Verification items for the finished model (mm, model axes). A direction names the side the tool comes from. Round coordinates to 2 decimals unless told otherwise and drop trailing zeros. Loops run counter-clockwise (first coordinate to the right, second up) from the corner with the lowest first, then second, coordinate; pieces in that order, holes last. Notation, with made-up numbers: (-3, 55) -> (20, 55) arc R36 ccw to (20, 91) -> close; hole circle Ø4 at (1, 25). An arc over 180 degrees is marked (long way). Write item = value, one per line. Start each with the question number.
```python
from build123d import *

# Parameters (mm, degrees)
F0_W     = 57.15
F0_H     = 44.45
F1_DEPTH = 25.4
F3_DEPTH = 12.7
F4_DEPTH = 19.05


with BuildPart() as f1:
    # F0 (on Front) → F1 (new body)
    with BuildSketch(Plane.XZ):
        with Locations((28.575, 22.225)):
            Rectangle(F0_W, F0_H)
    extrude(amount=F1_DEPTH)

    # F2 (on face) → F3 (cut)
    with BuildSketch(Plane.XZ.offset(25.4)):
        with BuildLine():
            Line((57.15, 44.45), (19.05, 44.45))
            Line((19.05, 44.45), (24.390971, 35.103302))
            ThreePointArc((24.390971, 35.103302), (41.651297, 30.339378), (36.992666, 13.050335))
            Line((36.992666, 13.050335), (44.45, 0))
            Line((44.45, 0), (57.15, 0))
            Line((57.15, 0), (57.15, 44.45))
        make_face()
    extrude(amount=-F3_DEPTH, mode=Mode.SUBTRACT)

    # F2 (on face) → F4 (cut)
    with BuildSketch(Plane.XZ.offset(25.4)):
        with BuildLine():
            ThreePointArc((36.992666, 13.050335), (41.651297, 30.339378), (24.390971, 35.103302))
            Line((24.390971, 35.103302), (36.992666, 13.050335))
        make_face()
        with BuildLine():
            Line((36.992666, 13.050335), (24.390971, 35.103302))
            ThreePointArc((24.390971, 35.103302), (19.597921, 17.737449), (36.992666, 13.050335))
        make_face()
    extrude(amount=-F4_DEPTH, mode=Mode.SUBTRACT)


solid = f1.part
```
(1) Section check C-C on y = -23. Enter the section's corners in (x, z), then the cut area to 3 significant figures.
(2) Depth check by flat-ended pin: pin 1 Ø1 at (x, z) = (36.5, 32.5) entering from -Y. Enter the tip coordinate at first touch or a pass-through.
(3) Scan lines: line 1 (Y direction, x = 27, z = 13.5); line 2 (Y direction, x = 51, z = 23); line 3 (Z direction, x = 24, y = -23). Record each from-to range of solid material in increasing order. Write a range as [from, to].
(4) Section check A-A on y = -12. Enter the section's corners in (x, z), then the cut area to 3 significant figures.
(5) Draft check along Z on faces 3 (the flat face through (57.15, -6, 22)), 4 (the flat face through (40.669, -19.139, 6.617)), 5 (the flat face through (30, -6.35, 24)), 6 (the flat face through (28, -13, 0)). Enter one of: +Z half, -Z half, draft (parallel to the pull), parting line (faces both ways), or undercut.
(6) Access from +Z, -Z, +X, -X, +Y, -Y to the whole of each face (thin tool, end or side, straight path). Record for faces 1 (the flat face through (0, -13, 22)), 2 (the flat face through (21.683, -19.139, 39.842)).
(7) Section check B-B on z = 3.5. Enter the section's corners in (x, y).
(8) Section check D-D on x = 30. Enter the section's corners in (y, z), then the cut area to 3 significant figures.
Computed values:
q1.outline = (0, 0) -> (44.45, 0) -> (36.99, 13.05) arc R12.7 cw (long way) to (24.39, 35.1) -> (19.05, 44.45) -> (0, 44.45) -> close
q1.area = 1,160 mm²
q2.pin_1 = -6.35
q3.line_1 = [-6.35, 0]
q3.line_2 = [-12.7, 0]
q3.line_3 = [0, 13.2], [34.87, 35.79]
q4.outline = (0, 0) -> (57.15, 0) -> (57.15, 44.45) -> (0, 44.45) -> close; hole circle Ø25.4 at (30.62, 24.04)
q4.area = 2,030 mm²
q5.face_3 = draft
q5.face_4 = +Z half
q5.face_5 = undercut
q5.face_6 = -Z half
q6.face_1 = +Z, -Z, -X, +Y, -Y
q6.face_2 = +Z, +X, -Y
q7.outline = (0, -25.4) -> (42.45, -25.4) -> (42.45, -12.7) -> (57.15, -12.7) -> (57.15, 0) -> (0, 0) -> close
q8.outline = (-25.4, 0) -> (0, 0) -> (0, 44.45) -> (-12.7, 44.45) -> (-12.7, 36.72) -> (-6.35, 36.72) -> (-6.35, 11.35) -> (-25.4, 11.35) -> close
q8.area = 548 mm²
